Here's the drawing with two shaded views (mm, measured from the low corner). I have some questions. A direction names the side the tool comes from. Coordinates: 2 decimals unless noted, no trailing zeros. Order: outer loops, then holes, each group sorted by start corner. A loop starts at its lowest first (then second) coordinate and runs counter-clockwise, first axis right, second up. Notation, with made-up numbers: (71, 0.25) -> (81, 0.25) arc R31 ccw to (81, 33.25) -> close; hole circle Ø9 at (78, 46). An arc over 180 degrees is marked (long way). Answer in a Markdown table with one row per item. Add a question column.
1. Imagine slicing it at D-D on x = 62. Write out the boundary of the cut face in (y, z) (1 decimal).
2. On a 3-axis mill with a long thin cutter (end or side, diameter ignored), from which of +Z, -Z, +X, -X, +Y, -Y can I reach the whole of each face in a straight line? I mean the marked faces 1 and 2. Say none if no direction works.
3. If I drill on line 1 along Z through (x, y) = (44.5, 1.75); line 2 along X through (y, z) = (9.25, 47.5); line 3 along Z through (x, y) = (70, 4.75) (1 decimal), over which ranges is the centre line in solid material (lowest first)? Write a range as [from, to].
4. Imagine slicing it at A-A on z = 45. Write out the boundary of the cut face in (x, y), plus the area to 3 significant figures.
5. We'd pull the mould along Z, two halves only. Please class the marked faces 3, 4, 5 and 6: pulls with the +Z half, pulls with the -Z half, needs draft (parallel to the pull), parting line crosses it, or undercut.
6. Imagine slicing it at C-C on y = 6.75. State how many separate pieces and enclosed holes the cut face has.
7. Will these pins go through, and if not, where does the flat tip stop? pin 1 (4 mm diameter, centred on x = 42, y = 7.5, fed in from -Z); pin 2 (5 mm diameter, centred on y = 6, z = 27.5, fed in from +X); pin 3 (1.5 mm diameter, centred on x = 70, y = 1.5, fed in from -Z); pin 4 (4 mm diameter, centred on x = 71.52, z = 71.52, fed in from -Y).
8. Imagine slicing it at B-B on x = 45. Write out the boundary of the cut face in (y, z).
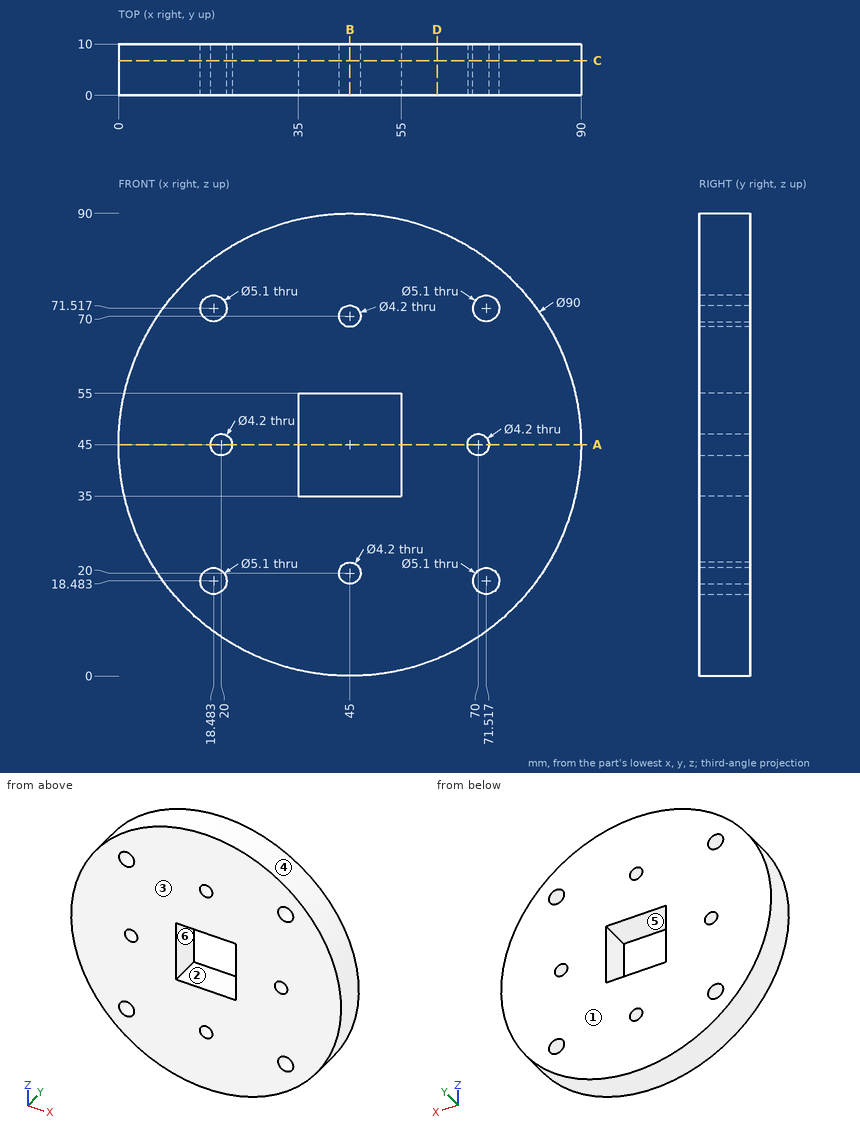
Answers follow:
| question | item | result |
|---|---|---|
| 1 | outline | (0, 3.3) -> (10, 3.3) -> (10, 86.7) -> (0, 86.7) -> close |
| 2 | face 1 | +Z, -Z, +X, -X, +Y |
| 2 | face 2 | +Y, -Y |
| 3 | line 1 | z = [0, 17.96], [22.04, 35], [55, 67.96], [72.04, 90] |
| 3 | line 2 | x = [0.07, 35], [55, 89.93] |
| 3 | line 3 | z = [7.6, 16.4], [20.5, 42.9], [47.1, 69.5], [73.6, 82.4] |
| 4 | outline | (0, 0) -> (17.9, 0) -> (17.9, 10) -> (0, 10) -> close; (22.1, 0) -> (35, 0) -> (35, 10) -> (22.1, 10) -> close; (55, 0) -> (67.9, 0) -> (67.9, 10) -> (55, 10) -> close; (72.1, 0) -> (90, 0) -> (90, 10) -> (72.1, 10) -> close |
| 4 | area | 616 mm² |
| 5 | face 3 | needs draft |
| 5 | face 4 | parting line crosses it |
| 5 | face 5 | undercut |
| 5 | face 6 | undercut |
| 6 | separate pieces | 1 |
| 6 | enclosed holes | 9 |
| 7 | pin 1 | stops at z = 0.01 |
| 7 | pin 2 | stops at x = 87.43 |
| 7 | pin 3 | stops at z = 7.09 |
| 7 | pin 4 | passes through |
| 8 | outline | (0, 0) -> (10, 0) -> (10, 17.9) -> (0, 17.9) -> close; (0, 22.1) -> (10, 22.1) -> (10, 35) -> (0, 35) -> close; (0, 55) -> (10, 55) -> (10, 67.9) -> (0, 67.9) -> close; (0, 72.1) -> (10, 72.1) -> (10, 90) -> (0, 90) -> close |
